Study the drawing (mm; zero at the part's minimum x, y, z) and answer. A direction names the side the tool comes from. Coordinates: 2 decimals unless noted, no trailing zeros. Loops run counter-clockwise (first coordinate to the right, second up) from the corner with the lowest first, then second, coordinate; pieces in that order, holes last. Notation, with made-up numbers: (-19, 12.25) -> (-9, 12.25) arc R29 cw to (-9, 39.25) -> close; hole circle Ø3 at (66, -19.75). An arc over 180 degrees is marked (long way). One line per question, with ' | ' between items. Start each with the question number.
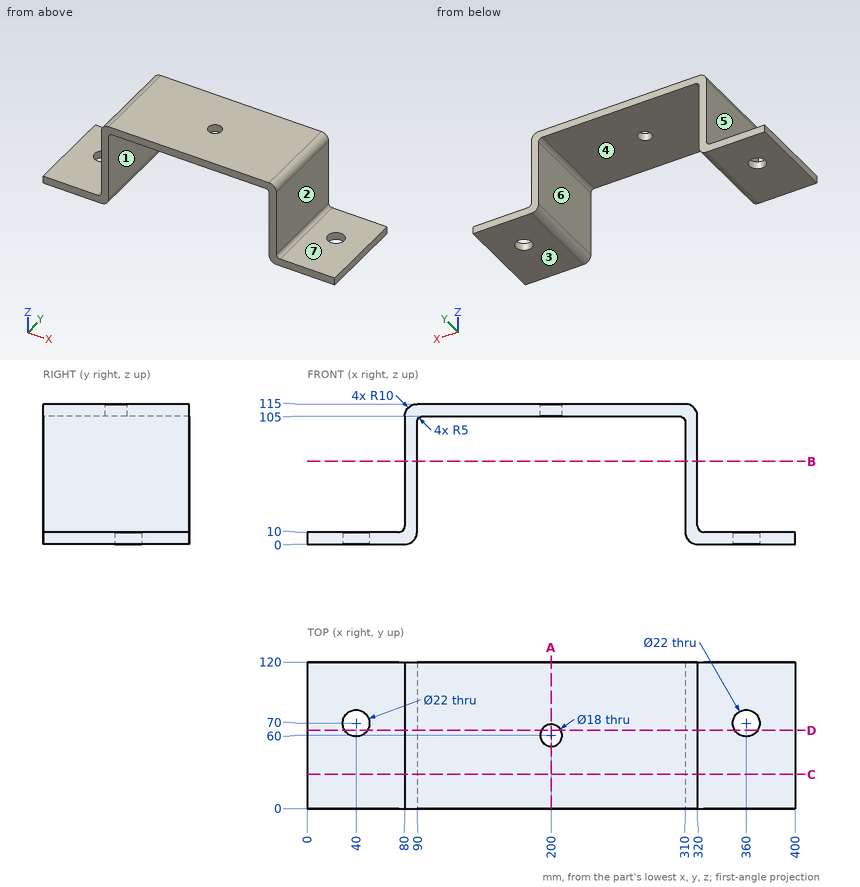
(1) Section A-A on x = 200 is taken. Write down the section's boundary in (y, z).
(2) Find the intervals of material crossed by probe 1 along Y at (x, z) = (200, 108.75); probe 2 along X at (y, z) = (96.5, 90); probe 3 along Y at (x, z) = (40, 3), in increasing order. Write a range as from..to.
(3) Section C-C on y = 28 is taken. Write down the section's boundary in (x, z).
(4) Section B-B on z = 68 is taken. Write down the section's boundary in (x, y), plus the area to 3 significant figures.
(5) Section D-D on y = 64 is taken. Give the number of separate pieces and of enclosed holes in the cut face, plus the area to 3 significant figures.
(6) Determine the mould class of the marked faces 1, 2, 3 and 4 for opening direction X: +X half, -X half, draft (parallel to the pull), parting line (faces both ways), or undercut.
(7) Each of these flat-tipped pins is pushed along its axis until it touches: pin 1 Ø5 at (y, z) = (91, 51.5) entering from -X; pin 2 Ø1.5 at (x, y) = (258.5, 69) entering from -Z; pin 3 Ø1 at (y, z) = (67, 72.5) entering from +X; pin 4 Ø10 at (x, z) = (302.5, 95) entering from -Y. Where does it stop, or does it pass through?
(8) A tool of negligible diameter and unlimited length cuts with its end or side. For the marked faces 5, 6 and 7, from which of +Z, -Z, +X, -X, +Y, -Y can it reach the whole face along a straight path? Write none if from no direction.
Working result:
1) outline: (0, 105) -> (51, 105) -> (51, 115) -> (0, 115) -> close; (69, 105) -> (120, 105) -> (120, 115) -> (69, 115) -> close
2) probe 1: y = 0..51, 69..120 | probe 2: x = 80..90, 310..320 | probe 3: y = 0..59, 81..120
3) outline: (0, 0) -> (80, 0) arc R10 ccw to (90, 10) -> (90, 100) arc R5 cw to (95, 105) -> (305, 105) arc R5 cw to (310, 100) -> (310, 10) arc R10 ccw to (320, 0) -> (400, 0) -> (400, 10) -> (325, 10) arc R5 cw to (320, 15) -> (320, 105) arc R10 ccw to (310, 115) -> (90, 115) arc R10 ccw to (80, 105) -> (80, 15) arc R5 cw to (75, 10) -> (0, 10) -> close
4) outline: (80, 0) -> (90, 0) -> (90, 120) -> (80, 120) -> close; (310, 0) -> (320, 0) -> (320, 120) -> (310, 120) -> close | area: 2,400 mm2
5) separate pieces: 4 | enclosed holes: 0 | area: 5,510 mm2
6) face 1: undercut | face 2: +X half | face 3: draft | face 4: undercut
7) pin 1: stops at x = 80 | pin 2: stops at z = 105 | pin 3: stops at x = 320 | pin 4: passes through
8) face 5: +Z, -X, +Y, -Y | face 6: -Z, +Y, -Y | face 7: +Z, +X, +Y, -Y
